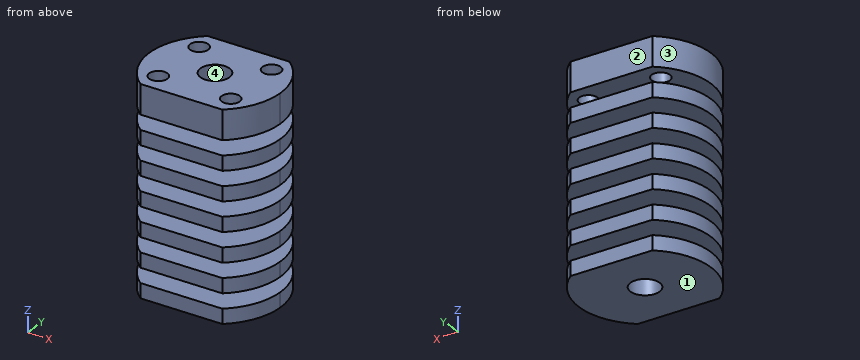
```python
from build123d import *

# Parameters (mm, degrees)
ESTRUSIONE_ESTRUSIONE1_DEPTH = 28
FORO_FILETTATO_M3_1_D        = 2.5
FORO_FILETTATO_M3_1_DEPTH    = 4.5
FORO_FILETTATO_M3_1_TIP      = 0.751075774
SCHIZZO4_R                   = 2
TAGLIO_ESTRUSIONE1_DEPTH     = 31.232432916
SCHIZZO5_W                   = 6
SCHIZZO5_H                   = 2
RIPETIZIONE_A_L1_COUNT       = 7
RIPETIZIONE_A_L1_PITCH       = 4


with BuildPart() as part:
    # Schizzo1 → Estrusione-Estrusione1 (new body)
    with BuildSketch(Plane.XY):
        with BuildLine():
            Line((5.656854249, 7), (-5.656854249, 7))
            ThreePointArc((-5.656854249, 7), (-9, 0), (-5.656854249, -7))
            Line((-5.656854249, -7), (5.656854249, -7))
            ThreePointArc((5.656854249, -7), (8.121320344, -3.878679656), (9, 0))
            ThreePointArc((9, 0), (8.121320344, 3.878679656), (5.656854249, 7))
        make_face()
    extrude(amount=ESTRUSIONE_ESTRUSIONE1_DEPTH)

    # Foro filettato M3-1
    with Locations(Plane(origin=(-5, 4.25, 28), x_dir=(1, 0, 0), z_dir=(0, 0, 1))):
        with Locations((0, 0), (10, 0), (0, -8.5), (10, -8.5)):
            Hole(FORO_FILETTATO_M3_1_D / 2, depth=FORO_FILETTATO_M3_1_DEPTH)
            with Locations((0, 0, -(FORO_FILETTATO_M3_1_DEPTH + FORO_FILETTATO_M3_1_TIP / 2))):  # 118° drill point
                Cone(0, FORO_FILETTATO_M3_1_D / 2, FORO_FILETTATO_M3_1_TIP, mode=Mode.SUBTRACT)

    # Schizzo4 → Taglio-Estrusione1 (cut, through all)
    with BuildSketch(Plane.XY.offset(28)):
        Circle(SCHIZZO4_R)
    extrude(amount=-TAGLIO_ESTRUSIONE1_DEPTH, mode=Mode.SUBTRACT)

    # Schizzo5 → Taglia-Rivoluzione1 (revolve, cut)
    with BuildSketch(Plane(origin=(0, 0, 0), x_dir=(1, 0, 0), z_dir=(0, 1, 0)), mode=Mode.PRIVATE) as taglia_rivoluzione1_sk:
        with Locations((6, -23)):
            Rectangle(SCHIZZO5_W, SCHIZZO5_H)
    taglia_rivoluzione1 = revolve(taglia_rivoluzione1_sk.sketch.rotate(Axis((0, 0, 0), (0, 0, 1)), 180), axis=Axis((0, 0, 0), (0, 0, 1)), mode=Mode.SUBTRACT)

    # Ripetizione a L1: Taglia-Rivoluzione1 ×7
    with Locations(*[(0, 0, -i * RIPETIZIONE_A_L1_PITCH) for i in range(1, RIPETIZIONE_A_L1_COUNT)]):
        add(taglia_rivoluzione1, mode=Mode.SUBTRACT)


solid = part.part
```
CAD build for the part. Positions are in the model's coordinates, mm. Face numbers are marked on the shaded views. Round coordinates to 2 decimals unless told otherwise and drop trailing zeros. Order: outer loops, then holes, each group sorted by start corner. A loop starts at its lowest first (then second) coordinate and runs counter-clockwise, first axis right, second up.
Item 1: Probe line 1 along Y through (x, z) = (5, 26.55); line 2 along Z through (x, y) = (-5.5, -4.25); line 3 along Y through (x, z) = (4, 25). List the from-to ranges inside material, lowest first.
Item 2: Saw through at A-A on x = 6.75. Write the cut outline in (y, z).
Item 3: Saw through at C-C on y = -6. Write the cut outline in (x, z), then the cut area to 3 significant figures.
Item 4: Mould opens along Y. For the marked faces 1, 2, 3 and 4 say: pulls with the +Y half, pulls with the -Y half, needs draft (parallel to the pull), parting line crosses it, or undercut.
Item 5: Pin check, flat tips, straight feed: pin 1 (3 mm diameter, centred on x = 5, y = -4.25, fed in from +Z); pin 2 (4 mm diameter, centred on y = 2.5, z = 14, fed in from +X); pin 3 (2 mm diameter, centred on x = 5, y = 4.25, fed in from +Z); pin 4 (4 mm diameter, centred on y = -4, z = 14.5, fed in from -X). Stop position of each tip, or through.
Item 6: Saw through at B-B on z = 9.5. Write the cut outline in (x, y).
Item 7: Saw through at D-D on x = -4.25. State how many separate pieces and enclosed holes the cut face has, then the cut area to 3 significant figures.
Reported:
1. line 1: y = -7 to -5.5, -3 to 3, 5.5 to 7
1. line 2: z = 0 to 2, 4 to 6, 8 to 10, 12 to 14, 16 to 18, 20 to 22
1. line 3: y = -7 to -5, -3.5 to 3.5, 5 to 7
2. outline: (-5.95, 0) - (5.95, 0) - (5.95, 2) - (-5.95, 2) - close; (-5.95, 4) - (5.95, 4) - (5.95, 6) - (-5.95, 6) - close; (-5.95, 8) - (5.95, 8) - (5.95, 10) - (-5.95, 10) - close; (-5.95, 12) - (5.95, 12) - (5.95, 14) - (-5.95, 14) - close; (-5.95, 16) - (5.95, 16) - (5.95, 18) - (-5.95, 18) - close; (-5.95, 20) - (5.95, 20) - (5.95, 22) - (-5.95, 22) - close; (-5.95, 24) - (5.95, 24) - (5.95, 28) - (-5.95, 28) - close
3. outline: (-6.71, 0) - (6.71, 0) - (6.71, 2) - (-6.71, 2) - close; (-6.71, 4) - (6.71, 4) - (6.71, 6) - (-6.71, 6) - close; (-6.71, 8) - (6.71, 8) - (6.71, 10) - (-6.71, 10) - close; (-6.71, 12) - (6.71, 12) - (6.71, 14) - (-6.71, 14) - close; (-6.71, 16) - (6.71, 16) - (6.71, 18) - (-6.71, 18) - close; (-6.71, 20) - (6.71, 20) - (6.71, 22) - (-6.71, 22) - close; (-6.71, 24) - (6.71, 24) - (6.71, 28) - (-6.71, 28) - close
3. area: 215 mm2
4. face 1: needs draft
4. face 2: pulls with the +Y half
4. face 3: parting line crosses it
4. face 4: undercut
5. pin 1: stops at z = 28
5. pin 2: stops at x = 8.99
5. pin 3: stops at z = 22
5. pin 4: stops at x = -8.76
6. outline: (-5.66, -7) - (5.66, -7) arc R9 ccw to (5.66, 7) - (-5.66, 7) arc R9 ccw to start; hole circle Ø4 at (0, 0)
7. separate pieces: 9
7. enclosed holes: 0
7. area: 208 mm2
